Source: CAD feature listing. Evaluate the final solid. Frame: model axes, mm. A direction names the side the tool comes from. Coordinates: 2 decimals unless noted, no trailing zeros. Write each loop counter-clockwise with the first axis right and the second up, starting at its lowest first coordinate (ties: lowest second). Pieces come first, ordered by that corner, then holes. Notation, with made-up numbers: M -28.75,56.5 L -19.75,56.5 A27 cw -19.75,73.5 Z; hole C 29,81 d10. An arc over 180 degrees is marked long. Answer as CSV lines item,"result". Start each with the question number.
1. Section C-C on z = 198.7. Return the cut outline in (x, y).
2. Section B-B on x = -208. Return the cut outline in (y, z).
3. Line query: probe 1 along X at (y, z) = (8.75, 210); probe 2 along Z at (x, y) = (-164, 10.75); probe 3 along X at (y, z) = (6, 156). Output: solid intervals per line, ascending. Write a range as [from, to].
4. Section A-A on z = 213.7. Return the cut outline in (x, y), plus the area to 3 significant figures.
5. Contact query for flat-ended pins moving along their axis: pin 1 Ø3.5 at (x, y) = (-201, 9) entering from +Z; pin 2 Ø6.5 at (x, y) = (-252, 3.5) entering from +Z; pin 3 Ø4 at (y, z) = (3.5, 218.5) entering from -X; pin 4 Ø8 at (x, z) = (-204, 189.5) entering from -Y. Output: stop coordinate, or through.
6. Mould query, pull axis Z, two halves, no side actions, for faces 5 (the face through (-210.447, 6, 217)), 6 (the face through (-151.924, 6.261, 198.542)), 7 (the face through (-198, 6, 210.5)). Classes: pulls with the +Z half, pulls with the -Z half, needs draft (parallel to the pull), parting line crosses it, or undercut.
7. Reachability of faces 1 (the face through (-160.157, 6, 220)), 2 (the face through (-245.03, 6.26, 86.89)), 3 (the face through (-235.447, 6, 217)), 4 (the face through (-254, 6, 170.5)) from +Z, -Z, +X, -X, +Y, -Y: full face, straight path, thin tool, end or side. Return the list, or none.
```python
from build123d import *

# Parameters (mm, degrees)
BOSS_EXTRUDE1_DEPTH = 12.7
SKETCH2_R           = 3.2
CUT_EXTRUDE1_DEPTH  = 344.457619003


with BuildPart() as part:
    # Sketch1 → Boss-Extrude1 (new body)
    with BuildSketch(Plane(origin=(0, 0, 0), x_dir=(1, 0, 0), z_dir=(0, 1, 0))):
        with BuildLine():
            Line((-134.869381255, -210.5), (-160.156660352, -210.5))
            Line((-160.156660352, -210.5), (-160.156660352, -223.2))
            Line((-160.156660352, -223.2), (-185.156660352, -223.2))
            Line((-185.156660352, -223.2), (-185.156660352, -210.5))
            Line((-185.156660352, -210.5), (-210.446660352, -210.5))
            Line((-210.446660352, -210.5), (-210.446660352, -223.2))
            Line((-210.446660352, -223.2), (-235.446660352, -223.2))
            Line((-235.446660352, -223.2), (-235.446660352, -210.5))
            Line((-235.446660352, -210.5), (-248.036660352, -210.5))
            Line((-248.036660352, -210.5), (-248.036660352, -195.5))
            Line((-248.036660352, -195.5), (-260.736660352, -195.5))
            Line((-260.736660352, -195.5), (-260.736660352, -170.5))
            Line((-260.736660352, -170.5), (-248.036660352, -170.5))
            Line((-248.036660352, -170.5), (-248.036660352, -125.974827547))
            Line((-248.036660352, -125.974827547), (-260.736660352, -125.974827547))
            Line((-260.736660352, -125.974827547), (-260.736660352, -100.974827547))
            Line((-260.736660352, -100.974827547), (-248.036660352, -100.974827547))
            Line((-248.036660352, -100.974827547), (-248.036660352, -85.974827547))
            Line((-248.036660352, -85.974827547), (-241.932414551, -87.830328326))
            Line((-241.932414551, -87.830328326), (-238.254147431, -75.729526817))
            ThreePointArc((-238.254147431, -75.729526817), (-215.223229772, -127.196546204), (-181.244243015, -172.193276216))
            Line((-181.244243015, -172.193276216), (-163.978062557, -154.927095758))
            Line((-163.978062557, -154.927095758), (-154.927095758, -163.978062557))
            Line((-154.927095758, -163.978062557), (-172.193276216, -181.244243015))
            ThreePointArc((-172.193276216, -181.244243015), (-154.226598654, -196.759132616), (-134.869381255, -210.5))
        make_face()
    extrude(amount=BOSS_EXTRUDE1_DEPTH)

    # Sketch2 → Cut-Extrude1 (cut, through all)
    with BuildSketch(Plane(origin=(0, 12.7, 0), x_dir=(1, 0, 0), z_dir=(0, 1, 0))):
        with Locations((-248.036660352, -129.174827547)):
            Circle(SKETCH2_R)
        with Locations((-248.036660352, -97.774827547)):
            Circle(SKETCH2_R)
        with Locations((-248.036660352, -167.3)):
            Circle(SKETCH2_R)
        with Locations((-248.036660352, -198.7)):
            Circle(SKETCH2_R)
        with Locations((-238.646660352, -210.5)):
            Circle(SKETCH2_R)
        with Locations((-207.246660352, -210.5)):
            Circle(SKETCH2_R)
        with Locations((-188.356660352, -210.5)):
            Circle(SKETCH2_R)
        with Locations((-160.156660352, -213.7)):
            Circle(SKETCH2_R)
        with Locations((-183.433424282, -169.859291345)):
            Circle(SKETCH2_R)
        with Locations((-169.859291345, -183.433424282)):
            Circle(SKETCH2_R)
        with Locations((-241.001759282, -84.768648922)):
            Circle(SKETCH2_R)
    extrude(amount=-CUT_EXTRUDE1_DEPTH, mode=Mode.SUBTRACT)


solid = part.part
```
Values:
1,outline,"M -244.84,0 L -151.72,0 L -151.72,12.7 L -244.84,12.7 Z"
2,outline,"M 0,138.69 L 12.7,138.69 L 12.7,207.39 L 0,207.39 Z"
3,probe 1,"[-248.04, -241.81], [-235.49, -210.41], [-204.09, -191.52], [-185.2, -135.65]"
3,probe 2,"[154.95, 173.05], [188.69, 223.2]"
3,probe 3,"[-248.04, -195.36], [-165.05, -162.91]"
4,outline,"M -235.45,0 L -210.45,0 L -210.45,12.7 L -235.45,12.7 Z; M -185.16,0 L -163.36,0 L -163.36,12.7 L -185.16,12.7 Z"
4,area,"594 mm²"
5,pin 1,"z = 210.5"
5,pin 2,"z = 195.5"
5,pin 3,"x = -235.45"
5,pin 4,"y = 0"
6,face 5,"needs draft"
6,face 6,"undercut"
6,face 7,"pulls with the +Z half"
7,face 1,"+Z, +X, +Y, -Y"
7,face 2,"-Z, +Y, -Y"
7,face 3,"+Z, -X, +Y, -Y"
7,face 4,"-X, +Y, -Y"
